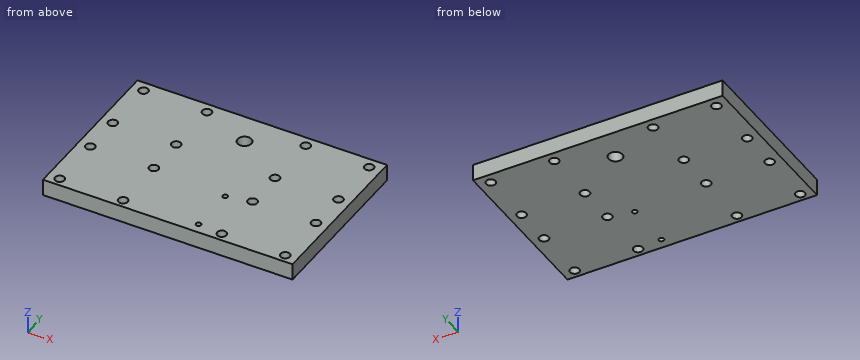
Autodesk Inventor part; units mm, degrees
ref_plane "YZ Plane" through (0, 0, 0) normal (1, 0, 0) x (0, 1, 0)
ref_plane "XZ Plane" through (0, 0, 0) normal (0, 1, 0) x (-1, 0, 0)
ref_plane "XY Plane" through (0, 0, 0) normal (0, 0, 1) x (1, 0, 0)
sketch "Sketch1" plane through (0, 0, 0) normal (0, 0, 1) x (1, 0, 0)
  line L0 (0, 0) -> (120, 0)
  line L1 (120, 0) -> (120, 80)
  line L2 (120, 80) -> (0, 80)
  line L3 (0, 80) -> (0, 0)
  dimension "width" = 120
  dimension "height" = 80
extrude "Extrusion1" add sketch "Sketch1" along normal blind 8
hole "Hole1" at (36.25, 75, 8) direction (0, 0, -1) diameter 4.5 end through all
pattern_linear "Rectangular Pattern1" count 2 spacing 30.5 along (-1, 0, 0) count 2 spacing 26 along (0, -1, 0) of "Hole1"
hole "Hole2" at (83.75, 75, 8) direction (0, 0, -1) diameter 4.5 end through all
pattern_linear "Rectangular Pattern2" count 2 spacing 30.5 along (1, 0, 0) count 2 spacing 26 along (0, -1, 0) of "Hole2"
pattern_linear "Rectangular Pattern3" count 2 spacing 45 along (0, -1, 0) of "Hole1", "Rectangular Pattern1", "Hole2", "Rectangular Pattern2"
hole "Hole3" at (60, 65, 8) direction (0, 0, -1) diameter 6.647 end through all
hole "Hole4" at (72, 5, 8) direction (0, 0, -1) diameter 2.459 end through all
hole "Hole5" at (72, 27.5, 8) direction (0, 0, -1) diameter 2.459 end through all
equation "\"d37\" = 0.5 * width"
properties part number "mobile plate"
Verification items for the finished model (mm, model axes). Coordinates: 2 decimals unless noted, no trailing zeros. Loops run counter-clockwise (first coordinate to the right, second up) from the corner with the lowest first, then second, coordinate; pieces in that order, holes last. Notation, with made-up numbers: (68.5, 19) -> (117.5, 19) arc R21 cw to (117.5, 49) -> close; hole circle Ø9 at (-11.5, -21). An arc over 180 degrees is marked (long way). Put each result on its own line as item: value.
1. Section check D-D, the plane z = 5.75. Give the number of separate pieces and of enclosed holes in the cut face, then the cut area to 3 significant figures.
Result set:
separate pieces: 1
enclosed holes: 19
area: 9,300 mm^2
2. Section check A-A, the plane y = 30. Record the boundary of the cut face in (x, z), then the cut area to 3 significant figures.
Result set:
outline: (0, 0) -> (3.5, 0) -> (3.5, 8) -> (0, 8) -> close; (8, 0) -> (34, 0) -> (34, 8) -> (8, 8) -> close; (38.5, 0) -> (81.5, 0) -> (81.5, 8) -> (38.5, 8) -> close; (86, 0) -> (112, 0) -> (112, 8) -> (86, 8) -> close; (116.5, 0) -> (120, 0) -> (120, 8) -> (116.5, 8) -> close
area: 816 mm^2
3. Section check C-C, the plane x = 36.25. Record the boundary of the cut face in (y, z), then the cut area to 3 significant figures.
Result set:
outline: (0, 0) -> (1.75, 0) -> (1.75, 8) -> (0, 8) -> close; (6.25, 0) -> (27.75, 0) -> (27.75, 8) -> (6.25, 8) -> close; (32.25, 0) -> (46.75, 0) -> (46.75, 8) -> (32.25, 8) -> close; (51.25, 0) -> (72.75, 0) -> (72.75, 8) -> (51.25, 8) -> close; (77.25, 0) -> (80, 0) -> (80, 8) -> (77.25, 8) -> close
area: 496 mm^2
4. Gauge pin test, flat ends, axial feed: P1, Ø3.5, axis at x = 5.75, y = 4, coming from the +Z side; P2, Ø7, axis at x = 5.75, y = 30, coming from the -Z side. Record the tip position at first contact, or that the pin passes through.
Result set:
P1: passes through
P2: stops at z = 0
5. Section check B-B, the plane x = 60. Record the boundary of the cut face in (y, z).
Result set:
outline: (0, 0) -> (61.68, 0) -> (61.68, 8) -> (0, 8) -> close; (68.32, 0) -> (80, 0) -> (80, 8) -> (68.32, 8) -> close
6. Thickness scan on line 1 (Y direction, x = 114.25, z = 2.25); line 2 (X direction, y = 75, z = 5.5); line 3 (X direction, y = 4, z = 3.25). Record the ranges inside material, lowest first.
Result set:
line 1: y = 0 to 1.75, 6.25 to 27.75, 32.25 to 46.75, 51.25 to 72.75, 77.25 to 80
line 2: x = 0 to 3.5, 8 to 34, 38.5 to 81.5, 86 to 112, 116.5 to 120
line 3: x = 0 to 3.5, 8 to 34, 38.5 to 71.28, 72.72 to 81.5, 86 to 112, 116.5 to 120
